```python
from build123d import *

# Parameters (mm, degrees)
SKETCH_W        = 20
SKETCH_H        = 20
SKETCH_R        = 1.6
PAD_DEPTH       = 3
PAD001_DEPTH    = 20
SKETCH002_R     = 1.6
POCKET_DEPTH    = 4.561
SKETCH003_W     = 20
SKETCH003_H     = 3
PAD002_DEPTH    = 12.5
SKETCH004_R     = 2.75
POCKET001_DEPTH = 5
SKETCH005_R     = 1.6
POCKET002_DEPTH = 20.001
FILLET_R        = 9
SKETCH006_W     = 5.5
SKETCH006_H     = 4.5
PAD003_DEPTH    = 3.5
POCKET003_DEPTH = 20.001


with BuildPart() as part:
    # Sketch → Pad (new body)
    with BuildSketch(Plane.XY):
        Rectangle(SKETCH_W, SKETCH_H)
        with Locations((0, -5.286)):
            Circle(SKETCH_R, mode=Mode.SUBTRACT)
        with Locations((0, 5.286)):
            Circle(SKETCH_R, mode=Mode.SUBTRACT)
    extrude(amount=PAD_DEPTH)

    # Sketch001 (on Face1 of Pad) → Pad001 (join)
    with BuildSketch(Plane(origin=(0, 10, 0), x_dir=(-1, 0, 0), z_dir=(0, 1, 0))):
        Polygon((0, 3), (-4.74, 3), (-2.94, 4.56), (2.94, 4.56), (4.74, 3), align=None)
    extrude(amount=-PAD001_DEPTH)

    # Sketch002 (on Face4 of Pad001) → Pocket (cut, through all)
    with BuildSketch(Plane(origin=(0, 0, 0), x_dir=(1, 0, 0), z_dir=(0, 0, -1))):
        with Locations((0, 5.286)):
            Circle(SKETCH002_R)
        with Locations((0, -5.286)):
            Circle(SKETCH002_R)
    extrude(amount=-POCKET_DEPTH, mode=Mode.SUBTRACT)

    # Sketch003 (on Face4 of Pocket) → Pad002 (join)
    with BuildSketch(Plane(origin=(0, 0, 0), x_dir=(1, 0, 0), z_dir=(0, 0, -1))):
        with Locations((0, 8.5)):
            Rectangle(SKETCH003_W, SKETCH003_H)
        with Locations((0, -8.5)):
            Rectangle(SKETCH003_W, SKETCH003_H)
    extrude(amount=PAD002_DEPTH)

    # Sketch004 (on Face10 of Pad002) → Pocket001 (cut)
    with BuildSketch(Plane(origin=(0, 0, 0), x_dir=(1, 0, 0), z_dir=(0, 0, -1))):
        with Locations((0, 5.286)):
            Circle(SKETCH004_R)
        with Locations((0, -5.286)):
            Circle(SKETCH004_R)
    extrude(amount=POCKET001_DEPTH, mode=Mode.SUBTRACT)

    # Sketch005 (on Face4 of Pocket001) → Pocket002 (cut, through all)
    with BuildSketch(Plane(origin=(0, 10, 0), x_dir=(-1, 0, 0), z_dir=(0, 1, 0))):
        with Locations((0, -8.25)):
            Circle(SKETCH005_R)
    extrude(amount=-POCKET002_DEPTH, mode=Mode.SUBTRACT)

    # Fillet
    fillet_edges = [part.edges().sort_by_distance(p)[0] for p in [
        (10, 8.5, -12.5),
        (-10, 8.5, -12.5),
        (10, -8.5, -12.5),
        (-10, -8.5, -12.5),
    ]]
    fillet(fillet_edges, radius=FILLET_R)

    # Sketch006 (on Face15 of Fillet) → Pad003 (join)
    with BuildSketch(Plane(origin=(0, 0, 0), x_dir=(1, 0, 0), z_dir=(0, 0, -1))):
        with Locations((-7.25, 4.75)):
            Rectangle(SKETCH006_W, SKETCH006_H)
        with Locations((-7.25, -4.75)):
            Rectangle(SKETCH006_W, SKETCH006_H)
        with Locations((7.25, 4.75)):
            Rectangle(SKETCH006_W, SKETCH006_H)
        with Locations((7.25, -4.75)):
            Rectangle(SKETCH006_W, SKETCH006_H)
    extrude(amount=PAD003_DEPTH)

    # Sketch007 (on Face9 of Pad003) → Pocket003 (cut, through all)
    with BuildSketch(Plane.YZ.offset(10)):
        Polygon((-2.5, 0), (-2.5, -3.5), (-7, -3.5), align=None)
        Polygon((7, -3.5), (2.5, -3.5), (2.5, 0), align=None)
    extrude(amount=-POCKET003_DEPTH, mode=Mode.SUBTRACT)


solid = part.part
```
Geometry check sheet. Reference: the model listing, model coordinates, mm. A direction names the side the tool comes from. Round coordinates to 2 decimals unless told otherwise and drop trailing zeros. Write each loop counter-clockwise with the first axis right and the second up, starting at its lowest first coordinate (ties: lowest second). Pieces come first, ordered by that corner, then holes. Notation, with made-up numbers: (37, 51) - (53, 51) arc R14 cw to (53, 70) - close; hole circle Ø1 at (-23, 63). An arc over 180 degrees is marked (long way). Write each question's results on one line, items separated by ' | '.
(1) Draft check along X on faces 6 (the face through (-10, 0, 1)), 7 (the face through (0.35, 8.52, -9.81)), 8 (the face through (7.294, -8.521, -9.934)), 9 (the face through (-4.5, 5, -1)). Enter one of: pulls with the +X half, pulls with the -X half, needs draft (parallel to the pull), parting line crosses it, or undercut.
Computed:
face 6: pulls with the -X half | face 7: undercut | face 8: pulls with the +X half | face 9: undercut
(2) Thickness scan on probe 1 along Y at (x, z) = (0, 2.8); probe 2 along Y at (x, z) = (3, -8.25); probe 3 along X at (y, z) = (-5.5, -0.5). Record the ranges inside material, lowest first. Write a range as from..to.
Computed:
probe 1: y = -10..-6.89, -3.69..3.69, 6.89..10 | probe 2: y = -10..-7, 7..10 | probe 3: x = -10..-4.5, 4.5..10
(3) Sectioned sample at D-D, the plane z = -0.5. Enter the section's corners in (x, y).
Computed:
outline: (-10, -10) - (10, -10) - (10, -3.14) - (4.5, -3.14) - (4.5, -7) - (2.15, -7) arc R2.75 cw to (-2.15, -7) - (-4.5, -7) - (-4.5, -3.14) - (-10, -3.14) - close; (-10, 3.14) - (-4.5, 3.14) - (-4.5, 7) - (-2.15, 7) arc R2.75 cw to (2.15, 7) - (4.5, 7) - (4.5, 3.14) - (10, 3.14) - (10, 10) - (-10, 10) - close
(4) Sectioned sample at C-C, the plane y = -6.25. Enter the section's corners in (x, z), plus the area to 3 significant figures.
Computed:
outline: (-10, -2.92) - (-4.5, -2.92) - (-4.5, 0) - (-1.28, 0) - (-1.28, 4.56) - (-2.94, 4.56) - (-4.74, 3) - (-10, 3) - close; (1.28, 0) - (4.5, 0) - (4.5, -2.92) - (10, -2.92) - (10, 3) - (4.74, 3) - (2.94, 4.56) - (1.28, 4.56) - close | area: 92.4 mm^2
(5) Set-up check for faces 1 (the face through (0, 7, -6)), 2 (the face through (0, 7.4, -5)), 3 (the face through (0, 8, -12.5)), 4 (the face through (-0.2, 3.7, 2.2)), 5 (the face through (7.288, -4.781, -1.774)): record each of +Z, -Z, +X, -X, +Y, -Y from which the full face is reachable in a straight line by a thin tool's end or side.
Computed:
face 1: -Z | face 2: none | face 3: -Z, +X, -X, +Y, -Y | face 4: +Z, -Z | face 5: -Z, +X, -X
(6) Sectioned sample at B-B, the plane z = -7.75. Enter the section's corners in (x, y).
Computed:
outline: (-8.93, -10) - (-1.52, -10) - (-1.52, -7) - (-8.93, -7) - close; (-8.93, 7) - (-1.52, 7) - (-1.52, 10) - (-8.93, 10) - close; (1.52, -10) - (8.93, -10) - (8.93, -7) - (1.52, -7) - close; (1.52, 7) - (8.93, 7) - (8.93, 10) - (1.52, 10) - close
(7) Depth check by flat-ended pin: pin 1 Ø5 at (x, y) = (7, -7) entering from +Z; pin 2 Ø1 at (x, y) = (5, 0.5) entering from -Z; pin 3 Ø3 at (x, y) = (-5, -5) entering from +Z. Enter the tip coordinate at first touch or a pass-through.
Computed:
pin 1: stops at z = 3.21 | pin 2: stops at z = 0 | pin 3: stops at z = 4.07
(8) Sectioned sample at A-A, the plane x = 0. Enter the section's corners in (y, z).
Computed:
outline: (-10, -12.5) - (-7, -12.5) - (-7, -9.85) - (-10, -9.85) - close; (-10, -6.65) - (-7, -6.65) - (-7, -5) - (-8.04, -5) - (-8.04, 0) - (-6.89, 0) - (-6.89, 4.56) - (-10, 4.56) - close; (-3.69, 0) - (3.69, 0) - (3.69, 4.56) - (-3.69, 4.56) - close; (6.89, 0) - (8.04, 0) - (8.04, -5) - (7, -5) - (7, -6.65) - (10, -6.65) - (10, 4.56) - (6.89, 4.56) - close; (7, -12.5) - (10, -12.5) - (10, -9.85) - (7, -9.85) - close
